from build123d import *

# Parameters (mm, degrees)
BOTTOM_PLATE_START     = -335.008892233
BOTTOM_PLATE_OUTLINE_W = 600
BOTTOM_PLATE_OUTLINE_H = 16
BOTTOM_PLATE_DEPTH     = 395
SKETCH1_W              = 315
SKETCH1_H              = 520
CUT_EXTRUDE1_DEPTH     = 516.485669921


# Read off the part's stored shape, not the designer's step: bottom-plate
with BuildPart() as part:
    # bottom-plate outline → bottom-plate (new body)
    with BuildSketch(Plane.YZ.offset(BOTTOM_PLATE_START)):
        with Locations((91.456917194, 326.460719179)):
            Rectangle(BOTTOM_PLATE_OUTLINE_W, BOTTOM_PLATE_OUTLINE_H)
    extrude(amount=BOTTOM_PLATE_DEPTH)

    # Sketch1 → Cut-Extrude1 (cut, through all)
    with BuildSketch(Plane.XY.offset(334.460719179)):
        with Locations((-137.508892233, 91.456917194)):
            Rectangle(SKETCH1_W, SKETCH1_H)
    extrude(amount=-CUT_EXTRUDE1_DEPTH, mode=Mode.SUBTRACT)


solid = part.part
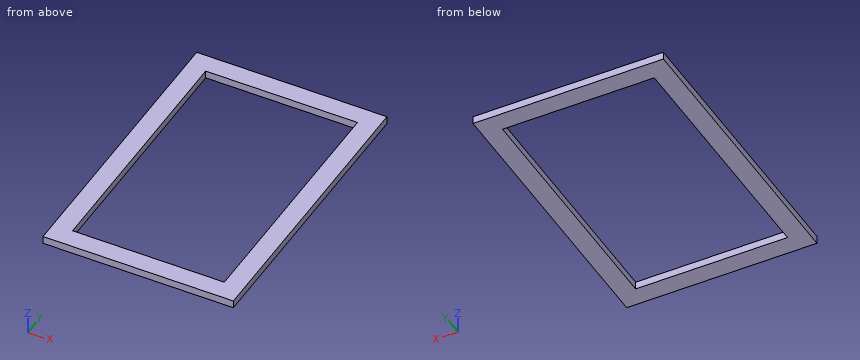
Geometry check sheet. Reference: the model listing, model coordinates, mm. Round coordinates to 2 decimals unless told otherwise and drop trailing zeros. Write each loop counter-clockwise with the first axis right and the second up, starting at its lowest first coordinate (ties: lowest second). Pieces come first, ordered by that corner, then holes. Notation, with made-up numbers: (28.5, -11.75) -> (33.5, -11.75) arc R7 ccw to (33.5, -1.75) -> close; hole circle Ø5 at (-8, 17). An arc over 180 degrees is marked (long way). One line per item, written item: value. Start each with the question number.
(1) Cross-section at A-A, the plane z = 332. Record the cut outline in (x, y), and give its area (3 significant figures).
(2) Scan lines: line 1 (X direction, y = 54, z = 330.75); line 2 (Y direction, x = -185, z = 326.75). Record each from-to range of solid material in increasing order. Write a range as [from, to].
(3) Cross-section at C-C, the plane x = -26.5. Record the cut outline in (y, z).
(4) Cross-section at B-B, the plane y = -10. Record the cut outline in (x, z), and give its area (3 significant figures).
Answer:
1. outline: (-335.01, -208.54) -> (59.99, -208.54) -> (59.99, 391.46) -> (-335.01, 391.46) -> close; hole (-295.01, -168.54) -> (19.99, -168.54) -> (19.99, 351.46) -> (-295.01, 351.46) -> close
1. area: 73,200 mm²
2. line 1: [-335.01, -295.01], [19.99, 59.99]
2. line 2: [-208.54, -168.54], [351.46, 391.46]
3. outline: (-208.54, 318.46) -> (-168.54, 318.46) -> (-168.54, 334.46) -> (-208.54, 334.46) -> close; (351.46, 318.46) -> (391.46, 318.46) -> (391.46, 334.46) -> (351.46, 334.46) -> close
4. outline: (-335.01, 318.46) -> (-295.01, 318.46) -> (-295.01, 334.46) -> (-335.01, 334.46) -> close; (19.99, 318.46) -> (59.99, 318.46) -> (59.99, 334.46) -> (19.99, 334.46) -> close
4. area: 1,280 mm²
